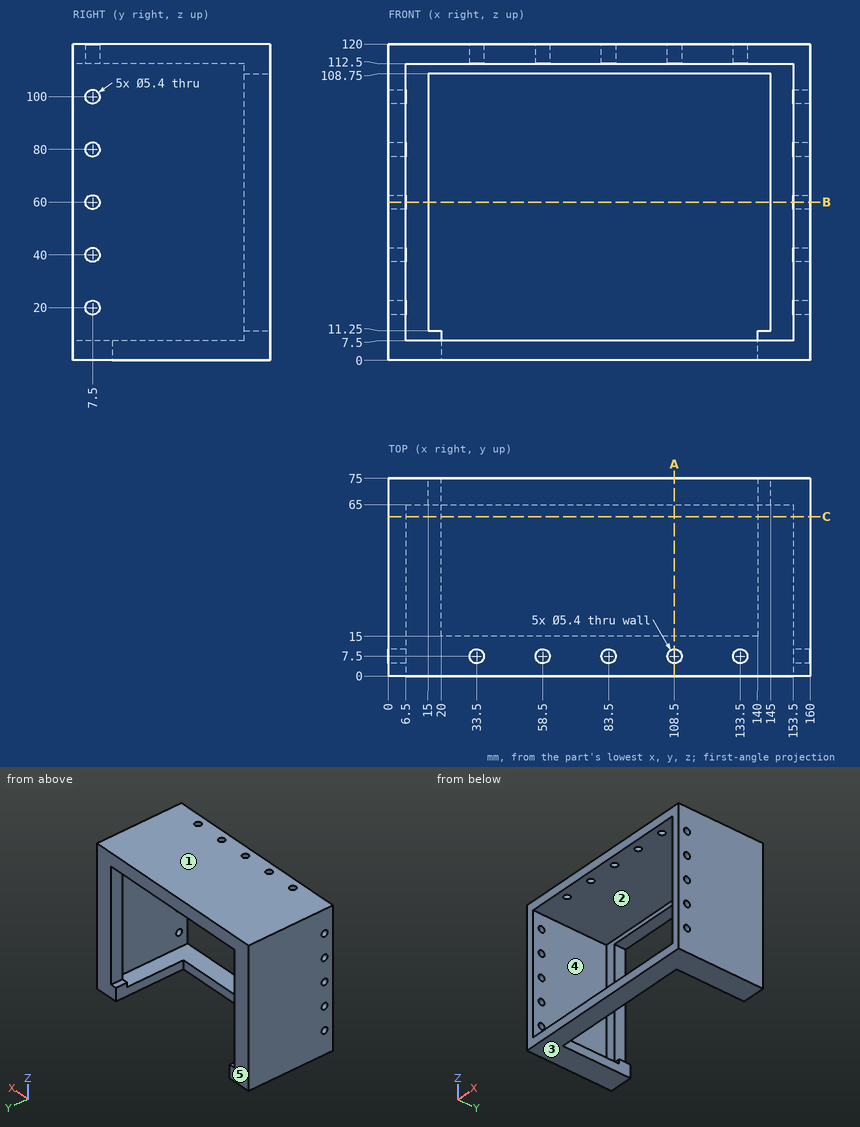
Input: dimensioned drawing with shaded views. Units: mm. Origin: part minimum x, y, z. A direction names the side the tool comes from. Give positions to 0.01 mm unless a question says otherwise; leave off trailing zeros. Loops run counter-clockwise (first coordinate to the right, second up) from the corner with the lowest first, then second, coordinate; pieces in that order, holes last. Notation, with made-up numbers: (24.5, 52.5) -> (36.5, 52.5) arc R21 ccw to (36.5, 85.5) -> close; hole circle Ø4 at (39, 0.25). An arc over 180 degrees is marked (long way). Use a Markdown table: item, result. Add a question column.
1) Section query B-B, the plane z = 60. Return the cut outline in (x, y), then the cut area to 3 significant figures.
2) Reachability of the marked faces 1 and 2 from +Z, -Z, +X, -X, +Y, -Y: full face, straight path, thin tool, end or side. Return the list, or none.
3) Section query C-C, the plane y = 60.5. Return the cut outline in (x, z), then the cut area to 4 significant figures.
4) Line query: line 1 along X through (y, z) = (4, 63); line 2 along X through (y, z) = (5.5, 115); line 3 along Z through (x, y) = (15, 30.5). Output: solid intervals per line, ascending. Write a range as [from, to].
5) Pull-direction query (Z, two-part tool) for the marked faces 3, 4 and 5; classes: +Z half, -Z half, draft (parallel to the pull), parting line (faces both ways), or undercut.
6) First-contact query: pin 1 (1 mm diameter, centred on x = 119.5, y = 43.5, fed in from -Z); pin 2 (6 mm diameter, centred on x = 77, z = 4.5, fed in from +Y). Flat tips, straight axial feed; report the tip coordinate or a pass-through.
7) Section query A-A, the plane x = 108.5. Return the cut outline in (y, z).
Numbers:
| question | item | result |
|---|---|---|
| 1 | outline | (0, 0) -> (6.5, 0) -> (6.5, 4.8) -> (0, 4.8) -> close; (0, 10.2) -> (6.5, 10.2) -> (6.5, 65) -> (15, 65) -> (15, 75) -> (0, 75) -> close; (145, 65) -> (153.5, 65) -> (153.5, 10.2) -> (160, 10.2) -> (160, 75) -> (145, 75) -> close; (153.5, 0) -> (160, 0) -> (160, 4.8) -> (153.5, 4.8) -> close |
| 1 | area | 1,070 mm2 |
| 2 | face 1 | +Z, +X, -X, +Y, -Y |
| 2 | face 2 | -Y |
| 3 | outline | (0, 0) -> (20, 0) -> (20, 7.5) -> (6.5, 7.5) -> (6.5, 112.5) -> (153.5, 112.5) -> (153.5, 7.5) -> (140, 7.5) -> (140, 0) -> (160, 0) -> (160, 120) -> (0, 120) -> close |
| 3 | area | 2,865 mm2 |
| 4 | line 1 | x = [0, 6.5], [153.5, 160] |
| 4 | line 2 | x = [0, 31.69], [35.31, 56.69], [60.31, 81.69], [85.31, 106.69], [110.31, 131.69], [135.31, 160] |
| 4 | line 3 | z = [0, 7.5], [112.5, 120] |
| 5 | face 3 | -Z half |
| 5 | face 4 | undercut |
| 5 | face 5 | draft |
| 6 | pin 1 | stops at z = 112.5 |
| 6 | pin 2 | stops at y = 15 |
| 7 | outline | (0, 0) -> (15, 0) -> (15, 7.5) -> (0, 7.5) -> close; (0, 112.5) -> (4.8, 112.5) -> (4.8, 120) -> (0, 120) -> close; (10.2, 112.5) -> (65, 112.5) -> (65, 108.75) -> (75, 108.75) -> (75, 120) -> (10.2, 120) -> close |
